For this review, take the finished solid that the model builds, in its own axes (mm). A direction names the side the tool comes from. Round coordinates to 2 decimals unless told otherwise and drop trailing zeros. Write each loop counter-clockwise with the first axis right and the second up, starting at its lowest first coordinate (ties: lowest second). Pieces come first, ordered by that corner, then holes.
from build123d import *

# Parameters (mm, degrees)
F1_DEPTH  = 12.7
F2_DEPTH  = 2.54
F3_DEPTH  = 7.62
F4_DEPTH  = 2.54
F5_DEPTH  = 2.54
F6_DEPTH  = 2.54
F7_DEPTH  = 2.54
F8_DEPTH  = 2.54
F9_DEPTH  = 2.54
F11_DEPTH = 10.16


with BuildPart() as f1:
    # F0 (on Front) → F1 (new body)
    with BuildSketch(Plane.XZ):
        Polygon((59.2296272516, 26.558874175), (0, 68.5641244054), (-54.7846257687, 26.558874175), (-54.7846257687, -40.5606217682), (0, -72.7868750691), (59.2296272516, -40.5606217682), align=None)
    extrude(amount=F1_DEPTH)

    # F2 (cut): a face of the model
    f2_faces = [f1.faces().sort_by_distance(p)[0] for p in [
        (1.9587071028, -12.7, -4.2659517496),
    ]]
    extrude(f2_faces, amount=-F2_DEPTH, mode=Mode.SUBTRACT)

    # F3 (cut): a face of the model
    f3_faces = [f1.faces().sort_by_distance(p)[0] for p in [
        (1.9587071028, -10.16, -4.2659517496),
    ]]
    extrude(f3_faces, amount=-F3_DEPTH, mode=Mode.SUBTRACT)

    # F4 (cut): a face of the model
    f4_faces = [f1.faces().sort_by_distance(p)[0] for p in [
        (29.6148136258, -1.27, 47.5614992902),
    ]]
    extrude(f4_faces, amount=-F4_DEPTH, mode=Mode.SUBTRACT)

    # F5 (cut): a face of the model
    f5_faces = [f1.faces().sort_by_distance(p)[0] for p in [
        (-27.3923128843, -1.27, 47.5614992902),
    ]]
    extrude(f5_faces, amount=-F5_DEPTH, mode=Mode.SUBTRACT)

    # F6 (cut): a face of the model
    f6_faces = [f1.faces().sort_by_distance(p)[0] for p in [
        (59.2296272516, -1.27, -7.0008737966),
    ]]
    extrude(f6_faces, amount=-F6_DEPTH, mode=Mode.SUBTRACT)

    # F7 (cut): a face of the model
    f7_faces = [f1.faces().sort_by_distance(p)[0] for p in [
        (-54.7846257687, -1.27, -7.0008737966),
    ]]
    extrude(f7_faces, amount=-F7_DEPTH, mode=Mode.SUBTRACT)

    # F8 (cut): a face of the model
    f8_faces = [f1.faces().sort_by_distance(p)[0] for p in [
        (-27.3923128843, -1.27, -56.6737484187),
    ]]
    extrude(f8_faces, amount=-F8_DEPTH, mode=Mode.SUBTRACT)

    # F9 (cut): a face of the model
    f9_faces = [f1.faces().sort_by_distance(p)[0] for p in [
        (29.6148136258, -1.27, -56.6737484187),
    ]]
    extrude(f9_faces, amount=-F9_DEPTH, mode=Mode.SUBTRACT)

    # F10 (on face) → F11 (join)
    with BuildSketch(Plane.XZ.offset(2.54)):
        Polygon((0, 23.3808644116), (-20.9086928517, -12.427886948), (20.4324796796, -12.3670902103), align=None)
        Polygon((-0.0592354809, -11.8803661317), (-9.8176104948, 5.073542241), (9.7081990615, 5.1022570899), align=None, mode=Mode.SUBTRACT)
    extrude(amount=F11_DEPTH)


solid = f1.part
(1) We need section D-D, the plane z = -35.5. Give the boundary of the cut face in (x, y).
Geometry check:
outline: (-52.24, -2.54) - (56.69, -2.54) - (56.69, 0) - (-52.24, 0) - close
(2) We need section B-B, the plane z = -5. Give the boundary of the cut face in (x, y), and give its area (3 significant figures).
Geometry check:
outline: (-52.24, -2.54) - (-16.57, -2.54) - (-16.57, -12.7) - (-4.02, -12.7) - (-4.02, -2.54) - (3.9, -2.54) - (3.9, -12.7) - (16.22, -12.7) - (16.22, -2.54) - (56.69, -2.54) - (56.69, 0) - (-52.24, 0) - close
area: 529 mm2
(3) We need section A-A, the plane y = -10. Give the boundary of the cut face in (x, z), and give its area (3 significant figures).
Geometry check:
outline: (-20.91, -12.43) - (20.43, -12.37) - (0, 23.38) - close; hole (-9.82, 5.07) - (-0.06, -11.88) - (9.71, 5.1) - close
area: 574 mm2
(4) Mouldability with a two-part tool opening along Z and no side actions: class faces 4 (the face through (-26.464, -1.252, -54.273)), 5 (the face through (-4.87, -7.55, -3.52)), 6 (the face through (10.359, -7.549, 5.257)) as pulls with the +Z half, pulls with the -Z half, needs draft (parallel to the pull), parting line crosses it, or undercut.
Geometry check:
face 4: pulls with the -Z half
face 5: undercut
face 6: pulls with the +Z half
(5) For faces 1 (the face through (4.893, -7.549, -3.27)), 2 (the face through (-10.308, -7.549, 5.727)), 3 (the face through (27.973, -1.252, -54.676)), list the 3-axis set-ups (+Z, -Z, +X, -X, +Y, -Y) from which the entire face can be reached by the end or side of a thin tool; tool diameter is ignored.
Geometry check:
face 1: -Y
face 2: +Z, -X, -Y
face 3: -Z, +X, +Y, -Y
(6) For pin 1 Ø6 at (x, y) = (-15, -1.5) entering from +Z; pin 2 Ø3 at (x, y) = (3, -10) entering from -Z; pin 3 Ø10 at (x, z) = (44, 41.5) entering from -Y, all flat-tipped, find the tip position at first contact; note any pin that passes through.
Geometry check:
pin 1: stops at z = 56.16
pin 2: stops at z = -12.39
pin 3: passes through
(7) We need section C-C, the plane x = -30.5. Give the boundary of the cut face in (y, z).
Geometry check:
outline: (-2.54, -51.9) - (0, -51.9) - (0, 41.98) - (-2.54, 41.98) - close
(8) For line 1 along Y through (x, z) = (17, -18.5); line 2 along Z through (x, y) = (-2.5, -10.25); line 3 along X through (y, z) = (-7, -10), list the stretches that pass through material, from the lowest coordinate up.
Geometry check:
line 1: y = -2.54 to 0
line 2: z = -12.4 to -7.64, 5.08 to 19.1
line 3: x = -19.49 to -1.14, 1.02 to 19.08
